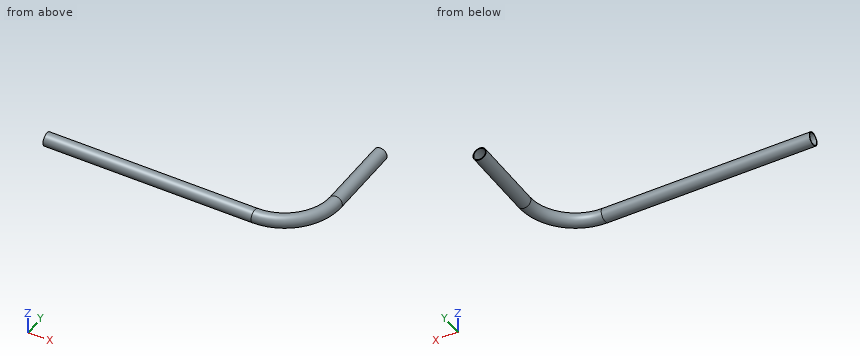
Autodesk Fusion 360 part; units mm, degrees
sketch "Sketch1" plane through (0, 0, 0) normal (1, 0, 0) x (0, 1, 0)
  circle A0 centre (0, 0) radius 1.3
  circle A1 centre (0, 0) radius 1.1476
  dimension "d1" = 2.6
  dimension "d2" = 2.2952
sketch "Sketch2" plane through (0, 0, 0) normal (0, 0, 1) x (1, 0, 0)
  line L0 (0, 0) -> (40.8, 0)
  line L1 (50.8, 10) -> (50.8, 25)
  arc A0 (40.8, 0) -> (50.8, 10) centre (40.8, 10) ccw
  point P0 (50.8, 0)
  dimension "d3" = 50.8
  dimension "d4" = 25
  dimension "d5" = 10
sweep "Sweep1" add profiles "Sketch1" path "Sketch2" along L0 A0 L1 section 1
equation "d2 = d1 - 0.012 in"
Work out the finished part from the listing and answer in its coordinate system (mm). Give positions to 0.01 mm unless a question says otherwise; leave off trailing zeros. Order: outer loops, then holes, each group sorted by start corner. A loop starts at its lowest first (then second) coordinate and runs counter-clockwise, first axis right, second up. Notation, with made-up numbers: (-31.5, -14.5) - (-8.5, -14.5) arc R9 cw to (-8.5, -2.5) - close; hole circle Ø11 at (-1.75, 28.25). An arc over 180 degrees is marked (long way). One line per item, written item: value. Start each with the question number.
1. Section C-C, the plane x = 19 is taken. Write down the section's boundary in (y, z).
2. Section B-B, the plane y = 19.25 is taken. Write down the section's boundary in (x, z), then the cut area to 3 significant figures.
3. This flat-tipped pin is pushed along its axis until it touches: pin 1 Ø1.5 at (y, z) = (1.5, -1) entering from +X. Where does it stop, or does it pass through?
4. Consider line 1 (Z direction, x = 24, y = 0); line 2 (X direction, y = 24, z = -0.4); line 3 (Y direction, x = 2.5, z = 0.2). Determine where each line is inside the solid, lowest interval first.
5. Section A-A, the plane z = 0 is taken. Write down the section's boundary in (x, y).
Filled sheet:
1. outline: circle Ø2.6 at (0, 0); hole circle Ø2.3 at (0, 0)
2. outline: circle Ø2.6 at (50.8, 0); hole circle Ø2.3 at (50.8, 0)
2. area: 1.17 mm²
3. pin 1: x = 48.71
4. line 1: -1.3 to -1.15, 1.15 to 1.3
4. line 2: 49.56 to 49.72, 51.88 to 52.04
4. line 3: -1.28 to -1.13, 1.13 to 1.28
5. outline: (0, -1.3) - (40.8, -1.3) arc R11.3 ccw to (52.1, 10) - (52.1, 25) - (51.95, 25) - (51.95, 10) arc R11.15 cw to (40.8, -1.15) - (0, -1.15) - close; (0, 1.15) - (40.8, 1.15) arc R8.85 ccw to (49.65, 10) - (49.65, 25) - (49.5, 25) - (49.5, 10) arc R8.7 cw to (40.8, 1.3) - (0, 1.3) - close
